Could you check a few things on this model? Use its own coordinates, in mm. Face numbers are marked on the shaded views. A direction names the side the tool comes from. Round coordinates to 2 decimals unless told otherwise and drop trailing zeros. Loops run counter-clockwise (first coordinate to the right, second up) from the corner with the lowest first, then second, coordinate; pieces in that order, holes last. Notation, with made-up numbers: M 4,-1.5 L 32,-1.5 A30 cw 32,20.5 Z; hole C 29,49 d5. An arc over 180 degrees is marked long. Answer in a Markdown table with one row per item.
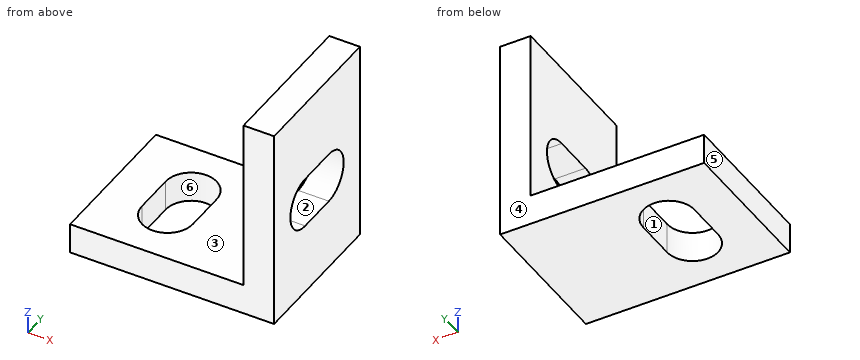
```python
from build123d import *

# Parameters (mm, degrees)
BOSS_EXTRUDE1_DEPTH     = 7.25
CUT_EXTRUDE1_DEPTH      = 18
CUT_EXTRUDE1_DEPTH_BACK = 4
CUT_EXTRUDE2_DEPTH      = 4
CUT_EXTRUDE2_DEPTH_BACK = 18


with BuildPart() as part:
    # Sketch1 → Boss-Extrude1 (new body, symmetric)
    with BuildSketch(Plane(origin=(0, 0, 0), x_dir=(1, 0, 0), z_dir=(0, 1, 0))):
        Polygon((0, 0), (0, -17), (3, -17), (3, 3), (-17, 3), (-17, 0), align=None)
    extrude(amount=BOSS_EXTRUDE1_DEPTH, both=True)

    # Sketch2 → Cut-Extrude1 (cut, two sides)
    with BuildSketch(Plane.XY) as cut_extrude1_sk:
        with BuildLine():
            Line((-8, 2), (-8, -2))
            ThreePointArc((-8, -2), (-10.5, -4.5), (-13, -2))
            Line((-13, -2), (-13, 2))
            ThreePointArc((-13, 2), (-10.5, 4.5), (-8, 2))
        make_face()
    extrude(amount=CUT_EXTRUDE1_DEPTH, mode=Mode.SUBTRACT)
    extrude(cut_extrude1_sk.sketch, amount=-CUT_EXTRUDE1_DEPTH_BACK, mode=Mode.SUBTRACT)

    # Sketch3 → Cut-Extrude2 (cut, two sides)
    with BuildSketch(Plane(origin=(0, 0, 0), x_dir=(0, 0, -1), z_dir=(1, 0, 0))) as cut_extrude2_sk:
        with BuildLine():
            Line((-4, 2), (-4, -2))
            ThreePointArc((-4, -2), (-6.5, -4.5), (-9, -2))
            Line((-9, -2), (-9, 2))
            ThreePointArc((-9, 2), (-6.5, 4.5), (-4, 2))
        make_face()
    extrude(amount=CUT_EXTRUDE2_DEPTH, mode=Mode.SUBTRACT)
    extrude(cut_extrude2_sk.sketch, amount=-CUT_EXTRUDE2_DEPTH_BACK, mode=Mode.SUBTRACT)


solid = part.part
```
1) Will these pins go through, and if not, where does the flat tip stop? P1, Ø4, axis at x = -2.5, y = 4.5, coming from the +Z side; P2, Ø8, axis at x = -3, y = -2.5, coming from the +Z side; P3, Ø8, axis at y = 4.5, z = 5, coming from the -X side.
Computed:
| item | result |
|---|---|
| P1 | stops at z = 0 |
| P2 | stops at z = 17 |
| P3 | stops at x = 0 |
2) I want a section at D-D, the plane z = -1. Please give me the cut outline in (x, y), plus the area to 3 significant figures.
Computed:
| item | result |
|---|---|
| outline | M -17,-7.25 L 3,-7.25 L 3,7.25 L -17,7.25 Z; hole M -13,-2 A2.5 ccw -8,-2 L -8,2 A2.5 ccw -13,2 Z |
| area | 250 mm² |
3) If we mould it in two halves opening along X, with no side actions, what happens to the marked faces 4, 5 and 6? For each: released by +X, released by -X, zero draft, split by the parting line, or undercut.
Computed:
| item | result |
|---|---|
| face 4 | zero draft |
| face 5 | released by -X |
| face 6 | undercut |
4) I want a section at A-A, the plane z = 6.5. Please give me the cut outline in (x, y).
Computed:
| item | result |
|---|---|
| outline | M 0,-7.25 L 3,-7.25 L 3,-4.5 L 0,-4.5 Z; M 0,4.5 L 3,4.5 L 3,7.25 L 0,7.25 Z |
5) I need wall thicknesses on line 1 (Z direction, x = -12, y = -6); line 2 (X direction, y = -4.75, z = 15); line 3 (Z direction, x = 2.25, y = 3.5). Which ranges of each line are inside material? Lowest first, please.
Computed:
| item | result |
|---|---|
| line 1 | z = -3 to 0 |
| line 2 | x = 0 to 3 |
| line 3 | z = -3 to 4.5, 8.5 to 17 |
6) I want a section at B-B, the plane x = -10.5. Please give me the cut outline in (y, z), plus the area to 3 significant figures.
Computed:
| item | result |
|---|---|
| outline | M -7.25,-3 L -4.5,-3 L -4.5,0 L -7.25,0 Z; M 4.5,-3 L 7.25,-3 L 7.25,0 L 4.5,0 Z |
| area | 16.5 mm² |
7) I want a section at C-C, the plane y = 1.5. Please give me the cut outline in (x, z), plus the area to 3 significant figures.
Computed:
| item | result |
|---|---|
| outline | M -17,-3 L -13,-3 L -13,0 L -17,0 Z; M -8,-3 L 3,-3 L 3,4 L 0,4 L 0,0 L -8,0 Z; M 0,9 L 3,9 L 3,17 L 0,17 Z |
| area | 81.0 mm² |
8) Which directions (+Z, -Z, +X, -X, +Y, -Y) give clear straight access to the entire face, cutting with the end or side of a thin tool? Please do the marked faces 1, 2 and 3.
Computed:
| item | result |
|---|---|
| face 1 | +Z, -Z |
| face 2 | +X, -X |
| face 3 | +Z, -X, +Y, -Y |
